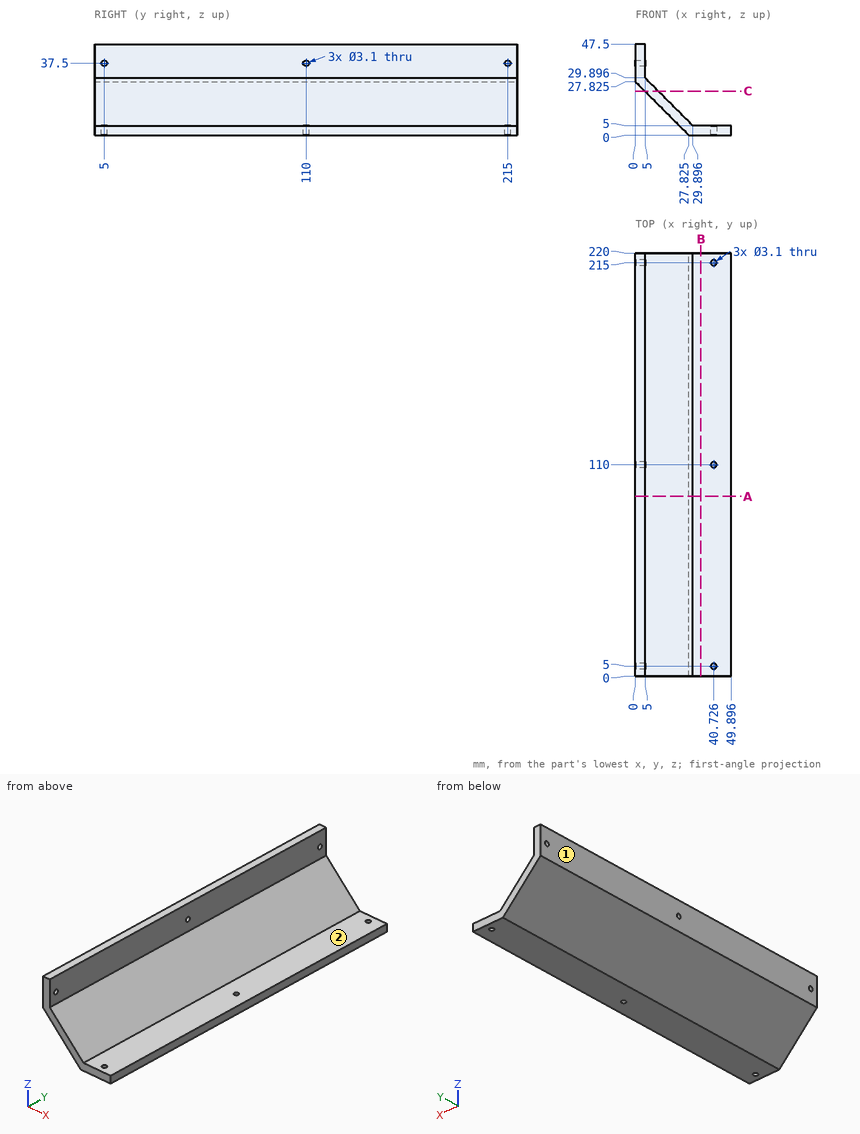
Check sheet for the drawn part. Datum: minimum x, y, z corner. Units: mm. A direction names the side the tool comes from. Round coordinates to 2 decimals unless told otherwise and drop trailing zeros. Order: outer loops, then holes, each group sorted by start corner. A loop starts at its lowest first (then second) coordinate and runs counter-clockwise, first axis right, second up. Notation, with made-up numbers: (64.25, 52) - (94.25, 52) arc R18 ccw to (94.25, 68) - close; hole circle Ø5 at (23.5, -5). An arc over 180 degrees is marked (long way). Use a Markdown table: item, result. Add a question column.
(1) Sectioned sample at B-B, the plane x = 34. Enter the section's corners in (y, z), and give its area (3 significant figures).
(2) Material ranges on line 1 along Z through (x, y) = (37.5, 204); line 2 along X through (y, z) = (110, 3.5) (1 decimal); line 3 along X through (y, z) = (215, 2.45) (1 decimal), recorded low to high. Write a range as [from, to].
(3) Depth check by flat-ended pin: pin 1 (5 mm diameter, centred on y = 52.5, z = 9, fed in from +X); pin 2 (1 mm diameter, centred on y = 87.5, z = 6.5, fed in from +X); pin 3 (10 mm diameter, centred on x = 42.5, y = 140.5, fed in from +Z). Enter the tip coordinate at first touch or a pass-through.
(4) Sectioned sample at C-C, the plane z = 23. Enter the section's corners in (x, y) (3 decimals), and give its area (3 significant figures).
(5) Sectioned sample at A-A, the plane y = 93.5. Enter the section's corners in (x, z) (3 decimals), and give its area (3 significant figures).
(6) Tool access check on the marked faces 1 and 2. Record the directions out of +Z, -Z, +X, -X, +Y, -Y that give a thin tool (end or side, any length) a straight path to the whole face; none if there is none.
Answers below:
| question | item | result |
|---|---|---|
| 1 | outline | (0, 0) - (220, 0) - (220, 5) - (0, 5) - close |
| 1 | area | 1,100 mm² |
| 2 | line 1 | [0, 5] |
| 2 | line 2 | [24.3, 39.2], [42.3, 49.9] |
| 2 | line 3 | [25.4, 39.2], [42.3, 49.9] |
| 3 | pin 1 | x = 28.4 |
| 3 | pin 2 | x = 28.9 |
| 3 | pin 3 | z = 5 |
| 4 | outline | (4.825, 0) - (11.896, 0) - (11.896, 220) - (4.825, 220) - close |
| 4 | area | 1,560 mm² |
| 5 | outline | (0, 27.825) - (27.825, 0) - (49.896, 0) - (49.896, 5) - (29.896, 5) - (5, 29.896) - (5, 47.5) - (0, 47.5) - close |
| 5 | area | 385 mm² |
| 6 | face 1 | +Z, -Z, -X, +Y, -Y |
| 6 | face 2 | +Z, +X, +Y, -Y |
